```python
from build123d import *

# Parameters (mm, degrees)
SKETCH1_R           = 9.5
BOSS_EXTRUDE1_DEPTH = 16
SKETCH1_3_R         = 10.75
SKETCH1_3_R_2       = 9.5
BOSS_EXTRUDE2_DEPTH = 11.5
SKETCH2_R           = 2
CUT_EXTRUDE1_DEPTH  = 23.070908454
SKETCH3_R           = 1.75
CUT_EXTRUDE2_DEPTH  = 23.070908454
CUT_EXTRUDE7_DEPTH  = 8
CUT_EXTRUDE8_DEPTH  = 6


with BuildPart() as part:
    # Sketch1 → Boss-Extrude1 (new body)
    with BuildSketch(Plane.XY):
        Circle(SKETCH1_R)
    extrude(amount=-BOSS_EXTRUDE1_DEPTH)

    # Sketch1_3 → Boss-Extrude2 (add)
    with BuildSketch(Plane.XY):
        Circle(SKETCH1_3_R)
        Circle(SKETCH1_3_R_2, mode=Mode.SUBTRACT)
    extrude(amount=-BOSS_EXTRUDE2_DEPTH)

    # Sketch2 → Cut-Extrude1 (cut, through all)
    with BuildSketch(Plane.XY):
        Circle(SKETCH2_R)
    extrude(amount=-CUT_EXTRUDE1_DEPTH, mode=Mode.SUBTRACT)

    # Sketch3 → Cut-Extrude2 (cut, through all)
    with BuildSketch(Plane(origin=(0, 0, -16), x_dir=(-1, 0, 0), z_dir=(0, 0, -1))):
        with Locations((0, 6.5)):
            Circle(SKETCH3_R)
        with Locations((-6.5, 0)):
            Circle(SKETCH3_R)
        with Locations((6.5, 0)):
            Circle(SKETCH3_R)
        with Locations((0, -6.5)):
            Circle(SKETCH3_R)
    extrude(amount=-CUT_EXTRUDE2_DEPTH, mode=Mode.SUBTRACT)

    # Sketch5 → Cut-Extrude7 (cut)
    with BuildSketch(Plane.XY):
        Polygon((1.58771324, 3.75), (3.175426481, 6.5), (1.58771324, 9.25), (-1.58771324, 9.25), (-3.175426481, 6.5), (-1.58771324, 3.75), align=None)
        Polygon((-4.91228676, -2.75), (-3.324573519, 0), (-4.91228676, 2.75), (-8.08771324, 2.75), (-9.675426481, 0), (-8.08771324, -2.75), align=None)
        Polygon((1.58771324, -9.25), (3.175426481, -6.5), (1.58771324, -3.75), (-1.58771324, -3.75), (-3.175426481, -6.5), (-1.58771324, -9.25), align=None)
        Polygon((8.08771324, -2.75), (9.675426481, 0), (8.08771324, 2.75), (4.91228676, 2.75), (3.324573519, 0), (4.91228676, -2.75), align=None)
    extrude(amount=-CUT_EXTRUDE7_DEPTH, mode=Mode.SUBTRACT)

    # Sketch6 → Cut-Extrude8 (cut)
    with BuildSketch(Plane.XY):
        Polygon((3.464101615, -6), (6.92820323, 0), (3.464101615, 6), (-3.464101615, 6), (-6.92820323, 0), (-3.464101615, -6), align=None)
    extrude(amount=-CUT_EXTRUDE8_DEPTH, mode=Mode.SUBTRACT)


solid = part.part
```
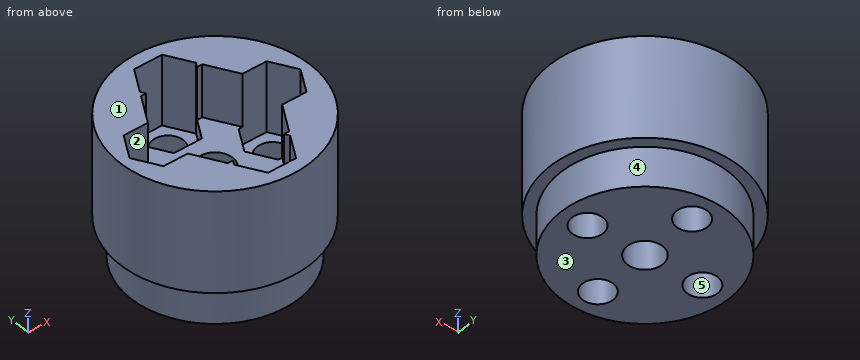
Geometry: final body of the model. Coordinates: model frame, mm. Face numbers are marked on the shaded views. A direction names the side the tool comes from. Round coordinates to 2 decimals unless told otherwise and drop trailing zeros. Write each loop counter-clockwise with the first axis right and the second up, starting at its lowest first coordinate (ties: lowest second). Pieces come first, ordered by that corner, then holes. Notation, with made-up numbers: M 14,47.25 L 50,47.25 A13 cw 50,68.25 Z; hole C 18,1.25 d4. An arc over 180 degrees is marked long. Answer in a Markdown table with one row per item. Add a question column.
(1) Draft query along X for the marked faces 3, 4 and 5. Return one class per face: pulls with the +X half, pulls with the -X half, needs draft (parallel to the pull), parting line crosses it, or undercut.
(2) Cut plane A-A, the plane x = 0. Return the cut outline in (y, z), then the cut area to 3 significant figures.
(3) Contact query for flat-ended pins moving along their axis: pin 1 (0.6 mm diameter, centred on x = 3, z = -3, fed in from -Y); pin 2 (1 mm diameter, centred on x = -7, z = -2.5, fed in from -Y); pin 3 (3 mm diameter, centred on y = 3, z = -8, fed in from -X); pin 4 (2 mm diameter, centred on x = -6.5, y = 0, fed in from -Z). Output: stop coordinate, or through.
(4) Cut plane C-C, the plane x = 6.75. Return the cut outline in (y, z), then the cut area to 3 significant figures.
(5) Reachability of the marked faces 1 and 2 from +Z, -Z, +X, -X, +Y, -Y: full face, straight path, thin tool, end or side. Return the list, or none.
(6) Cut plane D-D, the plane y = 7. Return the cut outline in (x, z).
(7) Cut plane B-B, the plane z = -10.75. Return the cut outline in (x, y), then the cut area to 3 significant figures.
(8) Ray query, L1, parallel to Y at x = 0, z = -13; L2, parallel to Y at x = -3, z = -5.25; L3, parallel to X at y = -0.75, z = -10. Return the intervals inside material, ascending.
Established:
| question | item | result |
|---|---|---|
| 1 | face 3 | needs draft |
| 1 | face 4 | parting line crosses it |
| 1 | face 5 | undercut |
| 2 | outline | M -10.75,-11.5 L -9.5,-11.5 L -9.5,-16 L -8.25,-16 L -8.25,-8 L -9.25,-8 L -9.25,0 L -10.75,0 Z; M -4.75,-16 L -2,-16 L -2,-6 L -3.75,-6 L -3.75,-8 L -4.75,-8 Z; M 2,-16 L 4.75,-16 L 4.75,-8 L 3.75,-8 L 3.75,-6 L 2,-6 Z; M 8.25,-16 L 9.5,-16 L 9.5,-11.5 L 10.75,-11.5 L 10.75,0 L 9.25,0 L 9.25,-8 L 8.25,-8 Z |
| 2 | area | 104 mm² |
| 3 | pin 1 | y = -10.41 |
| 3 | pin 2 | y = -8.56 |
| 3 | pin 3 | x = -10.64 |
| 3 | pin 4 | through |
| 4 | outline | M -8.37,-11.5 L -6.68,-11.5 L -6.68,-16 L -1.73,-16 L -1.73,-8 L -2.75,-8 L -2.75,0 L -8.37,0 Z; M 1.73,-16 L 6.68,-16 L 6.68,-11.5 L 8.37,-11.5 L 8.37,0 L 2.75,0 L 2.75,-8 L 1.73,-8 Z |
| 4 | area | 181 mm² |
| 5 | face 1 | +Z, +X, -X, +Y, -Y |
| 5 | face 2 | +Z |
| 6 | outline | M -8.16,-11.5 L -6.42,-11.5 L -6.42,-16 L -1.68,-16 L -1.68,-8 L -2.89,-8 L -2.89,0 L -8.16,0 Z; M 1.68,-16 L 6.42,-16 L 6.42,-11.5 L 8.16,-11.5 L 8.16,0 L 2.89,0 L 2.89,-8 L 1.68,-8 Z |
| 7 | outline | C 0,0 d21.5; hole C -6.5,0 d3.5; hole C 0,0 d4; hole C 0,-6.5 d3.5; hole C 0,6.5 d3.5; hole C 6.5,0 d3.5 |
| 7 | area | 312 mm² |
| 8 | L1 | -9.5 to -8.25, -4.75 to -2, 2 to 4.75, 8.25 to 9.5 |
| 8 | L2 | -10.32 to -6.8, -6.2 to -6, 6 to 6.2, 6.8 to 10.32 |
| 8 | L3 | -10.72 to -8.08, -4.92 to -1.85, 1.85 to 4.92, 8.08 to 10.72 |
